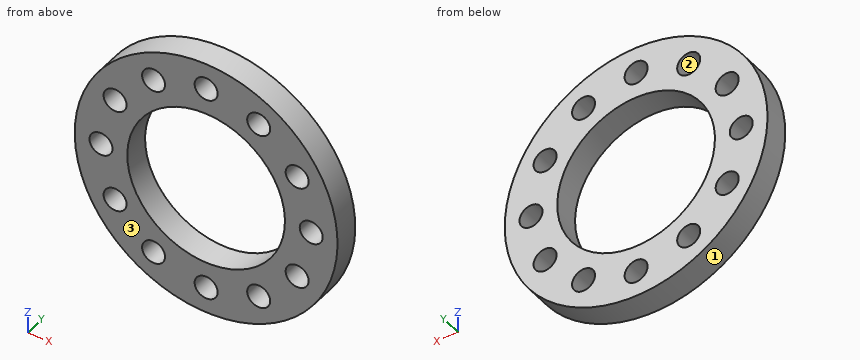
```python
from build123d import *

# Parameters (mm, degrees)
ESBO_O1_R                = 20
ESBO_O1_R_2              = 1.75
ESBO_O1_R_3              = 12
RESSALTO_EXTRUS_O1_DEPTH = 4


with BuildPart() as part:
    # Esboço1 → Ressalto-extrusão1 (new body)
    with BuildSketch(Plane(origin=(0, 0, 0), x_dir=(1, 0, 0), z_dir=(0, 1, 0))):
        with Locations(Location((0, 0, 0), (0, 0, 270))):
            Circle(ESBO_O1_R)
        with Locations(Location((0, 16, 0), (0, 0, 270))):
            Circle(ESBO_O1_R_2, mode=Mode.SUBTRACT)
        with Locations(Location((8, 13.856406461, 0), (0, 0, 270))):
            Circle(ESBO_O1_R_2, mode=Mode.SUBTRACT)
        with Locations(Location((13.856406461, 8, 0), (0, 0, 270))):
            Circle(ESBO_O1_R_2, mode=Mode.SUBTRACT)
        with Locations(Location((16, 0, 0), (0, 0, 270))):
            Circle(ESBO_O1_R_2, mode=Mode.SUBTRACT)
        with Locations(Location((13.856406461, -8, 0), (0, 0, 270))):
            Circle(ESBO_O1_R_2, mode=Mode.SUBTRACT)
        with Locations(Location((0, -16, 0), (0, 0, 270))):
            Circle(ESBO_O1_R_2, mode=Mode.SUBTRACT)
        with Locations(Location((8, -13.856406461, 0), (0, 0, 270))):
            Circle(ESBO_O1_R_2, mode=Mode.SUBTRACT)
        with Locations(Location((-8, -13.856406461, 0), (0, 0, 270))):
            Circle(ESBO_O1_R_2, mode=Mode.SUBTRACT)
        with Locations(Location((-13.856406461, -8, 0), (0, 0, 270))):
            Circle(ESBO_O1_R_2, mode=Mode.SUBTRACT)
        with Locations(Location((-16, 0, 0), (0, 0, 270))):
            Circle(ESBO_O1_R_2, mode=Mode.SUBTRACT)
        with Locations(Location((-13.856406461, 8, 0), (0, 0, 270))):
            Circle(ESBO_O1_R_2, mode=Mode.SUBTRACT)
        with Locations(Location((-8, 13.856406461, 0), (0, 0, 270))):
            Circle(ESBO_O1_R_2, mode=Mode.SUBTRACT)
        with Locations(Location((0, 0, 0), (0, 0, 270))):
            Circle(ESBO_O1_R_3, mode=Mode.SUBTRACT)
    extrude(amount=RESSALTO_EXTRUS_O1_DEPTH)


solid = part.part
```
Geometry check sheet. Reference: the model listing, model coordinates, mm. Face numbers are marked on the shaded views. Coordinates: 2 decimals unless noted, no trailing zeros. Write each loop counter-clockwise with the first axis right and the second up, starting at its lowest first coordinate (ties: lowest second). Pieces come first, ordered by that corner, then holes. Notation, with made-up numbers: M 20,-14 L 67,-14 A11 cw 67,-6 Z; hole C 30.5,37.25 d6. An arc over 180 degrees is marked long. Use one line per item in the form item = value. Start each with the question number.
1) Thickness scan on probe 1 along X at (y, z) = (2.05, -16); probe 2 along Z at (x, y) = (-1, 2.7); probe 3 along X at (y, z) = (1.4, -7) (3 decimals). Record the ranges inside material, lowest first. Write a range as from..to.
2) Go/stop test with flat-tipped pins: pin 1 Ø2 at (y, z) = (1, -5.5) entering from -X; pin 2 Ø1.5 at (y, z) = (1.5, 6.5) entering from +X. Record where each tip stops, or that it passes through.
3) Section check C-C on y = 1.2. State how many separate pieces and enclosed holes the cut face has, and give its area (3 significant figures).
4) Release check for a two-part mould opening along Z. For the marked faces 1, 2 and 3 record: pulls with the +Z half, pulls with the -Z half, needs draft (parallel to the pull), parting line crosses it, or undercut.
5) Section check A-A on z = -8. Enter the section's corners in (x, y).
6) Section check B-B on x = -13. Enter the section's corners in (y, z), and give its area (3 significant figures).
7) Section check D-D on x = 10.5. Enter the section's corners in (y, z).
Responses:
q1.probe_1 = -12..-1.75, 1.75..12
q1.probe_2 = -19.97..-17.44, -14.56..-11.96, 11.96..14.56, 17.44..19.97
q1.probe_3 = -18.735..-15.293, -12.42..-9.747, 9.747..12.42, 15.293..18.735
q2.pin_1 = -19.49
q2.pin_2 = 19.16
q3.separate_pieces = 1
q3.enclosed_holes = 13
q3.area = 689 mm2
q4.face_1 = parting line crosses it
q4.face_2 = undercut
q4.face_3 = needs draft
q5.outline = M -18.33,0 L -15.61,0 L -15.61,4 L -18.33,4 Z; M -12.11,0 L -8.94,0 L -8.94,4 L -12.11,4 Z; M 8.94,0 L 12.11,0 L 12.11,4 L 8.94,4 Z; M 15.61,0 L 18.33,0 L 18.33,4 L 15.61,4 Z
q6.outline = M 0,-15.2 L 4,-15.2 L 4,-9.53 L 0,-9.53 Z; M 0,-6.47 L 4,-6.47 L 4,6.47 L 0,6.47 Z; M 0,9.53 L 4,9.53 L 4,15.2 L 0,15.2 Z
q6.area = 97.2 mm2
q7.outline = M 0,-17.02 L 4,-17.02 L 4,-5.81 L 0,-5.81 Z; M 0,5.81 L 4,5.81 L 4,17.02 L 0,17.02 Z
